Could you check a few things on this model? Use its own coordinates, in mm. A direction names the side the tool comes from. Round coordinates to 2 decimals unless told otherwise and drop trailing zeros. Order: outer loops, then holes, each group sorted by start corner. A loop starts at its lowest first (then second) coordinate and runs counter-clockwise, first axis right, second up.
```python
from build123d import *

# Parameters (mm, degrees)
SKETCH_1_W          = 32.4
SKETCH_1_H          = 12
EXTRUDE_1_DEPTH     = 10
SKETCH_4_R          = 4
CUT_EXTRUDE_2_DEPTH = 8.5
SKETCH_7_R          = 3.4
CUT_EXTRUDE_3_DEPTH = 7.9
SKETCH_8_R          = 4.5
CUT_EXTRUDE_4_DEPTH = 16


with BuildPart() as part:
    # 草圖1 → 填料-伸長1 (new body)
    with BuildSketch(Plane(origin=(0, 0, 0), x_dir=(1, 0, 0), z_dir=(0, 1, 0))):
        Rectangle(SKETCH_1_W, SKETCH_1_H)
    extrude(amount=EXTRUDE_1_DEPTH)

    # 草圖4 → 除料-伸長2 (cut)
    with BuildSketch(Plane.ZY.offset(16.2)):
        with Locations((0, 7)):
            Circle(SKETCH_4_R)
    extrude(amount=-CUT_EXTRUDE_2_DEPTH, mode=Mode.SUBTRACT)

    # 草圖7 → 除料-伸長3 (cut)
    with BuildSketch(Plane.ZY.offset(7.7)):
        with Locations((0, 7)):
            Circle(SKETCH_7_R)
    extrude(amount=-CUT_EXTRUDE_3_DEPTH, mode=Mode.SUBTRACT)

    # 草圖8 → 除料-伸長4 (cut)
    with BuildSketch(Plane(origin=(16.2, 0, 0), x_dir=(0, 0, -1), z_dir=(1, 0, 0))):
        with Locations((0, 7)):
            Circle(SKETCH_8_R)
    extrude(amount=-CUT_EXTRUDE_4_DEPTH, mode=Mode.SUBTRACT)


solid = part.part
```
Q1. We'd pull the mould along Y, two halves only. Please class faces 4 (the flat face through (16.2, 2, 0)), 5 (the cylindrical face through (-12, 3, 0)), 6 (the flat face through (0, 10, -4)): released by +Y, released by -Y, zero draft, split by the parting line, or undercut.
Q2. Imagine slicing it at D-D, the plane x = 6.5. Please give me the cut outline in (y, z).
Q3. For P1, Ø2, axis at x = 7.5, z = 1.5, coming from the +Y side; P2, Ø4, axis at x = 6.5, z = -2, coming from the +Y side, each with a flat end and sliding along its axis, tell me the tip position at first contact or that it passes through.
Q4. Imagine slicing it at B-B, the plane z = 0. Please give me the cut outline in (x, y), then the cut area to 3 significant figures.
Q5. Imagine slicing it at A-A, the plane y = 7. Please give me the cut outline in (x, z).
Q6. For faces 1 (the flat face through (0, 0, 0)), 2 (the flat face through (0.2, 3, 0)), 3 (the flat face through (-7.7, 4, -2)), which set-ups out of +Z, -Z, +X, -X, +Y, -Y let a thin tool reach every point of the face, with its end or its side?
Q7. Imagine slicing it at C-C, the plane z = 2. Please give me the cut outline in (x, y).
Q8. I need wall thicknesses on L1, parallel to Z at x = 4.25, y = 7; L2, parallel to Y at x = 4.75, z = 0; L3, parallel to Y at x = -4, z = -2.75. Which ranges of each line are inside material? Lowest first, please.
Filled in:
1. face 4: zero draft
1. face 5: undercut
1. face 6: released by +Y
2. outline: (0, -6) - (10, -6) - (10, -3.35) arc R4.5 cw (long way) to (10, 3.35) - (10, 6) - (0, 6) - close
3. P1: stops at y = 3.26
3. P2: stops at y = 10
4. outline: (-16.2, 0) - (16.2, 0) - (16.2, 2.5) - (0.2, 2.5) - (0.2, 3.6) - (-7.7, 3.6) - (-7.7, 3) - (-16.2, 3) - close
4. area: 93.9 mm2
5. outline: (-16.2, -6) - (16.2, -6) - (16.2, -4.5) - (0.2, -4.5) - (0.2, -3.4) - (-7.7, -3.4) - (-7.7, -4) - (-16.2, -4) - close; (-16.2, 4) - (-7.7, 4) - (-7.7, 3.4) - (0.2, 3.4) - (0.2, 4.5) - (16.2, 4.5) - (16.2, 6) - (-16.2, 6) - close
6. face 1: +Z, -Z, +X, -X, -Y
6. face 2: +X
6. face 3: -X
7. outline: (-16.2, 0) - (16.2, 0) - (16.2, 2.97) - (0.2, 2.97) - (0.2, 4.25) - (-7.7, 4.25) - (-7.7, 3.54) - (-16.2, 3.54) - close; (-7.7, 9.75) - (0.2, 9.75) - (0.2, 10) - (-7.7, 10) - close
8. L1: z = -6 to -4.5, 4.5 to 6
8. L2: y = 0 to 2.5
8. L3: y = 0 to 5, 9 to 10
